```python
from build123d import *

# Parameters (mm, degrees)
BOSS_EXTRU_1_DEPTH = 5


with BuildPart() as part:
    # Esquisse1 → Boss.-Extru.1 (new body)
    with BuildSketch(Plane.XY):
        with BuildLine():
            Line((-10, 0), (-10, -42.679491924))
            Line((-10, -42.679491924), (-15, -42.679491924))
            Line((-15, -42.679491924), (-15, -69.679491924))
            Line((-15, -69.679491924), (-20, -69.679491924))
            Line((-20, -69.679491924), (-20, -74.679491924))
            Line((-20, -74.679491924), (-25, -74.679491924))
            Line((-25, -74.679491924), (-25, -42.679491924))
            Line((-25, -42.679491924), (-28.5, -42.679491924))
            Line((-28.5, -42.679491924), (-28.5, -39.679491924))
            Line((-28.5, -39.679491924), (-27.4, -39.679491924))
            Line((-27.4, -39.679491924), (-27.4, -37.379491924))
            Line((-27.4, -37.379491924), (-28.5, -37.379491924))
            Line((-28.5, -37.379491924), (-28.5, -32.679491924))
            Line((-28.5, -32.679491924), (-31.5, -32.679491924))
            Line((-31.5, -32.679491924), (-31.5, -37.379491924))
            Line((-31.5, -37.379491924), (-32.6, -37.379491924))
            Line((-32.6, -37.379491924), (-32.6, -39.679491924))
            Line((-32.6, -39.679491924), (-31.5, -39.679491924))
            Line((-31.5, -39.679491924), (-31.5, -42.679491924))
            Line((-31.5, -42.679491924), (-35, -42.679491924))
            Line((-35, -42.679491924), (-35, -69.679491924))
            Line((-35, -69.679491924), (-40, -69.679491924))
            Line((-40, -69.679491924), (-40, -74.679491924))
            Line((-40, -74.679491924), (-45, -74.679491924))
            Line((-45, -74.679491924), (-45, -69.679491924))
            Line((-45, -69.679491924), (-48.5, -69.679491924))
            Line((-48.5, -69.679491924), (-48.5, -66.679491924))
            Line((-48.5, -66.679491924), (-47.4, -66.679491924))
            Line((-47.4, -66.679491924), (-47.4, -64.379491924))
            Line((-47.4, -64.379491924), (-48.5, -64.379491924))
            Line((-48.5, -64.379491924), (-48.5, -59.679491924))
            Line((-48.5, -59.679491924), (-51.5, -59.679491924))
            Line((-51.5, -59.679491924), (-51.5, -64.379491924))
            Line((-51.5, -64.379491924), (-52.6, -64.379491924))
            Line((-52.6, -64.379491924), (-52.6, -66.679491924))
            Line((-52.6, -66.679491924), (-51.5, -66.679491924))
            Line((-51.5, -66.679491924), (-51.5, -69.679491924))
            Line((-51.5, -69.679491924), (-55, -69.679491924))
            Line((-55, -69.679491924), (-55, -74.679491924))
            Line((-55, -74.679491924), (-60, -74.679491924))
            Line((-60, -74.679491924), (-60, -69.679491924))
            Line((-60, -69.679491924), (-65, -69.679491924))
            Line((-65, -69.679491924), (-65, -42.679491924))
            Line((-65, -42.679491924), (-70, -42.679491924))
            Line((-70, -42.679491924), (-70, 25.320508076))
            ThreePointArc((-70, 25.320508076), (-61.213203436, 46.533711511), (-40, 55.320508076))
            Line((-40, 55.320508076), (-5, 55.320508076))
            ThreePointArc((-5, 55.320508076), (-1.464466094, 53.856041982), (0, 50.320508076))
            Line((0, 50.320508076), (0, 45.320508076))
            Line((0, 45.320508076), (5, 45.320508076))
            Line((5, 45.320508076), (5, 40.320508076))
            Line((5, 40.320508076), (0, 40.320508076))
            Line((0, 40.320508076), (0, 36.820508076))
            Line((0, 36.820508076), (-3, 36.820508076))
            Line((-3, 36.820508076), (-3, 37.920508076))
            Line((-3, 37.920508076), (-5.3, 37.920508076))
            Line((-5.3, 37.920508076), (-5.3, 36.820508076))
            Line((-5.3, 36.820508076), (-10, 36.820508076))
            Line((-10, 36.820508076), (-10, 33.820508076))
            Line((-10, 33.820508076), (-5.3, 33.820508076))
            Line((-5.3, 33.820508076), (-5.3, 32.720508076))
            Line((-5.3, 32.720508076), (-3, 32.720508076))
            Line((-3, 32.720508076), (-3, 33.820508076))
            Line((-3, 33.820508076), (0, 33.820508076))
            Line((0, 33.820508076), (0, 30.320508076))
            Line((0, 30.320508076), (5, 30.320508076))
            Line((5, 30.320508076), (5, 25.320508076))
            Line((5, 25.320508076), (0, 25.320508076))
            Line((0, 25.320508076), (0, 17.320508076))
            ThreePointArc((0, 17.320508076), (-1.339745962, 12.320508076), (-5, 8.660254038))
            ThreePointArc((-5, 8.660254038), (-8.660254038, 5), (-10, 0))
        make_face()
    extrude(amount=BOSS_EXTRU_1_DEPTH)


solid = part.part
```
Verification items for the finished model (mm, model axes). A direction names the side the tool comes from. Round coordinates to 2 decimals unless told otherwise and drop trailing zeros. Order: outer loops, then holes, each group sorted by start corner. A loop starts at its lowest first (then second) coordinate and runs counter-clockwise, first axis right, second up. Notation, with made-up numbers: (39, -24) -> (71, -24) arc R34 ccw to (71, 10) -> close; hole circle Ø8 at (68.25, -26.5). An arc over 180 degrees is marked (long way). Put each result on its own line as item: value. Start each with the question number.
(1) Tool access check on faces 1 (the face through (-42, -74.679, 2)), 2 (the face through (-33, -42.679, 2)), 3 (the face through (-20, -72, 2)), 4 (the face through (-27.4, -39, 2)), 5 (the face through (2, 30.321, 2)). Record the directions out of +Z, -Z, +X, -X, +Y, -Y that give a thin tool (end or side, any length) a straight path to the whole face; none if there is none.
(2) Section check B-B (y = 12). Enter the section's corners in (x, z).
(3) Depth check by flat-ended pin: pin 1 Ø2.5 at (y, z) = (-71, 2.5) entering from +X; pin 2 Ø2.5 at (x, z) = (-17, 3) entering from -Y; pin 3 Ø1.5 at (x, z) = (-26, 2) entering from -Y; pin 4 Ø4 at (x, y) = (-32.5, -52) entering from +Z. Enter the tip coordinate at first touch or a pass-through.
(4) Draft check along X on faces 6 (the face through (-60, -72, 2)), 7 (the face through (-4, 32.721, 2)), 8 (the face through (-67, -42.679, 2)), 9 (the face through (-31.5, -35, 2)). Enter one of: +X half, -X half, draft (parallel to the pull), parting line (faces both ways), or undercut.
(5) Material ranges on line 1 along X through (y, z) = (-69, 2.75); line 2 along X through (y, z) = (-65, 0.5); line 3 along Y through (x, z) = (-32.5, 3), recorded low to high.
(6) Section check A-A (y = -20). Enter the section's corners in (x, z).
Completed:
1. face 1: +Z, -Z, +X, -X, -Y
1. face 2: +Z, -Z, -Y
1. face 3: +Z, -Z, +X, -Y
1. face 4: +Z, -Z
1. face 5: +Z, -Z, +X
2. outline: (-70, 0) -> (-1.53, 0) -> (-1.53, 5) -> (-70, 5) -> close
3. pin 1: stops at x = -20
3. pin 2: stops at y = -69.68
3. pin 3: stops at y = -42.68
3. pin 4: passes through
4. face 6: -X half
4. face 7: undercut
4. face 8: draft
4. face 9: undercut
5. line 1: x = -65 to -51.5, -48.5 to -35, -25 to -15
5. line 2: x = -65 to -52.6, -47.4 to -35, -25 to -15
5. line 3: y = -42.68 to -39.68, -37.38 to 55.32
6. outline: (-70, 0) -> (-10, 0) -> (-10, 5) -> (-70, 5) -> close
